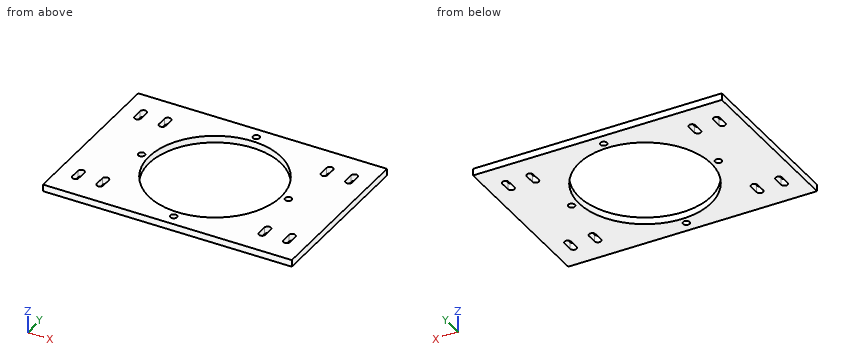
from build123d import *

# Parameters (mm, degrees)
SKETCH1_W                                = 152.4
SKETCH1_H                                = 138.176
SKETCH1_R                                = 53.975
BOSS_EXTRUDE1_DEPTH                      = 5.588
SKETCH5_R                                = 2.665
CUT_EXTRUDE4_DEPTH                       = 450.319819698
CUT_EXTRUDE5_DEPTH                       = 104.008822379
MIRROR1_AT_THE_SECOND_PLANE_COPY_1_DEPTH = 104.008822379
SKETCH7_W                                = 5.588
SKETCH7_H                                = 138.176
BOSS_EXTRUDE2_DEPTH                      = 25.4
CUT_EXTRUDE6_DEPTH                       = 123.991615519
MIRROR3_COPY_1_DEPTH                     = 123.991615519
SKETCH9_R                                = 2.7
CUT_EXTRUDE7_DEPTH                       = 483.750396617


with BuildPart() as part:
    # Sketch1 → Boss-Extrude1 (new body)
    with BuildSketch(Plane.XY):
        Rectangle(SKETCH1_W, SKETCH1_H)
        Circle(SKETCH1_R, mode=Mode.SUBTRACT)
    extrude(amount=BOSS_EXTRUDE1_DEPTH)

    # Sketch5 → Cut-Extrude4 (cut, through all)
    with BuildSketch(Plane(origin=(-338.200209725, -104.490630048, 5.588), x_dir=(0.9999190535665993, -0.012723455288419956, 0), z_dir=(0, 0, 1))):
        with Locations(Location((403.626134832, 63.40628164, 0), (0, 0, 0.729019959))):
            Circle(SKETCH5_R)
    extrude(amount=-CUT_EXTRUDE4_DEPTH, mode=Mode.SUBTRACT)

    # Sketch6 → Cut-Extrude5 (cut, through all)
    with BuildSketch(Plane(origin=(0, 0, 0), x_dir=(-1, 0, 0), z_dir=(0, 0, -1))):
        with BuildLine():
            Line((-68.865, -49.163584611), (-68.865, -41.163584611))
            ThreePointArc((-68.865, -41.163584611), (-66.2, -38.498584611), (-63.535, -41.163584611))
            Line((-63.535, -41.163584611), (-63.535, -49.163584611))
            ThreePointArc((-63.535, -49.163584611), (-66.2, -51.828584611), (-68.865, -49.163584611))
        make_face()
    cut_extrude5 = extrude(amount=-CUT_EXTRUDE5_DEPTH, mode=Mode.SUBTRACT)

    # Mirror1: Cut-Extrude5 across plane
    add(cut_extrude5.mirror(Plane(origin=(0, 0, 0), x_dir=(0, 0, 1), z_dir=(1, 0, 0))), mode=Mode.SUBTRACT)

    # Mirror1 at the second plane: Cut-Extrude5 across plane
    add(cut_extrude5.mirror(Plane.ZX), mode=Mode.SUBTRACT)

    # Mirror1 at the second plane copy 1 sketc → Mirror1 at the second plane copy 1 (cut, through all)
    with BuildSketch(Plane(origin=(0, 0, 0), x_dir=(1, 0, 0), z_dir=(0, 0, -1))):
        with BuildLine():
            Line((-68.865, -49.163584611), (-68.865, -41.163584611))
            ThreePointArc((-68.865, -41.163584611), (-66.2, -38.498584611), (-63.535, -41.163584611))
            Line((-63.535, -41.163584611), (-63.535, -49.163584611))
            ThreePointArc((-63.535, -49.163584611), (-66.2, -51.828584611), (-68.865, -49.163584611))
        make_face()
    extrude(amount=-MIRROR1_AT_THE_SECOND_PLANE_COPY_1_DEPTH, mode=Mode.SUBTRACT)

    # Sketch7 → Boss-Extrude2 (add)
    with BuildSketch(Plane(origin=(76.2, 0, 0), x_dir=(0, 0, -1), z_dir=(1, 0, 0))):
        with Locations((-2.794, 0)):
            Rectangle(SKETCH7_W, SKETCH7_H)
    boss_extrude2 = extrude(amount=BOSS_EXTRUDE2_DEPTH)

    # Sketch8 → Cut-Extrude6 (cut, through all)
    with BuildSketch(Plane(origin=(0, 0, 0), x_dir=(-1, 0, 0), z_dir=(0, 0, -1))):
        with BuildLine():
            Line((-63.535, 49.163584611), (-63.535, 41.163584611))
            ThreePointArc((-63.535, 41.163584611), (-66.2, 38.498584611), (-68.865, 41.163584611))
            Line((-68.865, 41.163584611), (-68.865, 49.163584611))
            ThreePointArc((-68.865, 49.163584611), (-66.2, 51.828584611), (-63.535, 49.163584611))
        make_face()
        with BuildLine():
            Line((-83.535, 41.163584611), (-83.535, 49.163584611))
            ThreePointArc((-83.535, 49.163584611), (-86.2, 51.828584611), (-88.865, 49.163584611))
            Line((-88.865, 49.163584611), (-88.865, 41.163584611))
            ThreePointArc((-88.865, 41.163584611), (-86.2, 38.498584611), (-83.535, 41.163584611))
        make_face()
    cut_extrude6 = extrude(amount=-CUT_EXTRUDE6_DEPTH, mode=Mode.SUBTRACT)

    # Mirror2: Cut-Extrude6 across plane
    add(cut_extrude6.mirror(Plane.ZX), mode=Mode.SUBTRACT)

    # Mirror3: Boss-Extrude2, Cut-Extrude6 across plane
    add(boss_extrude2.mirror(Plane(origin=(0, 0, 0), x_dir=(0, 0, 1), z_dir=(1, 0, 0))))
    add(cut_extrude6.mirror(Plane(origin=(0, 0, 0), x_dir=(0, 0, 1), z_dir=(1, 0, 0))), mode=Mode.SUBTRACT)

    # Mirror3 copy 1 sketch → Mirror3 copy 1 (cut, through all)
    with BuildSketch(Plane(origin=(0, 0, 0), x_dir=(1, 0, 0), z_dir=(0, 0, -1))):
        with BuildLine():
            Line((-63.535, 49.163584611), (-63.535, 41.163584611))
            ThreePointArc((-63.535, 41.163584611), (-66.2, 38.498584611), (-68.865, 41.163584611))
            Line((-68.865, 41.163584611), (-68.865, 49.163584611))
            ThreePointArc((-68.865, 49.163584611), (-66.2, 51.828584611), (-63.535, 49.163584611))
        make_face()
        with BuildLine():
            Line((-83.535, 41.163584611), (-83.535, 49.163584611))
            ThreePointArc((-83.535, 49.163584611), (-86.2, 51.828584611), (-88.865, 49.163584611))
            Line((-88.865, 49.163584611), (-88.865, 41.163584611))
            ThreePointArc((-88.865, 41.163584611), (-86.2, 38.498584611), (-83.535, 41.163584611))
        make_face()
    extrude(amount=-MIRROR3_COPY_1_DEPTH, mode=Mode.SUBTRACT)

    # Sketch9 → Cut-Extrude7 (cut, through all)
    with BuildSketch(Plane(origin=(-338.200209725, -129.890630048, 0), x_dir=(-0.9999190535665993, 0.012723455288419956, 0), z_dir=(0, 0, -1))):
        with Locations(Location((-276.525032787, 133.419783795, 0), (0, 0, 359.270980041))):
            Circle(SKETCH9_R)
        with Locations(Location((-337.283583318, 74.188047898, 0), (0, 0, 359.270980041))):
            Circle(SKETCH9_R)
        with Locations(Location((-396.515319215, 134.946598429, 0), (0, 0, 359.270980041))):
            Circle(SKETCH9_R)
        with Locations(Location((-335.756768683, 194.178334326, 0), (0, 0, 359.270980041))):
            Circle(SKETCH9_R)
    extrude(amount=-CUT_EXTRUDE7_DEPTH, mode=Mode.SUBTRACT)


solid = part.part
Verification items for the finished model (mm, model axes). Coordinates: 2 decimals unless noted, no trailing zeros. Loops run counter-clockwise (first coordinate to the right, second up) from the corner with the lowest first, then second, coordinate; pieces in that order, holes last. Notation, with made-up numbers: (5, 80) -> (34, 80) arc R24 ccw to (34, 95) -> close; hole circle Ø6 at (70.25, 6). An arc over 180 degrees is marked (long way). Answer as CSV lines item,"result".
1) Cross-section at B-B, the plane y = -60. Record the cut outline in (x, z), then the cut area to 3 significant figures.
Found:
outline,"(-101.6, 0) -> (-2.7, 0) -> (-2.7, 5.59) -> (-101.6, 5.59) -> close; (2.7, 0) -> (101.6, 0) -> (101.6, 5.59) -> (2.7, 5.59) -> close"
area,"1,110 mm2"
2) Cross-section at D-D, the plane y = 0. Record the cut outline in (x, z) (3 decimals).
Found:
outline,"(-101.6, 0) -> (-62.7, 0) -> (-62.7, 5.588) -> (-101.6, 5.588) -> close; (-57.3, 0) -> (-53.975, 0) -> (-53.975, 5.588) -> (-57.3, 5.588) -> close; (53.975, 0) -> (57.3, 0) -> (57.3, 5.588) -> (53.975, 5.588) -> close; (62.7, 0) -> (101.6, 0) -> (101.6, 5.588) -> (62.7, 5.588) -> close"
3) Cross-section at A-A, the plane x = 0. Record the cut outline in (y, z) (3 decimals), then the cut area to 3 significant figures.
Found:
outline,"(-69.088, 0) -> (-62.7, 0) -> (-62.7, 5.588) -> (-69.088, 5.588) -> close; (-57.3, 0) -> (-53.975, 0) -> (-53.975, 5.588) -> (-57.3, 5.588) -> close; (53.975, 0) -> (57.3, 0) -> (57.3, 5.588) -> (53.975, 5.588) -> close; (62.7, 0) -> (69.088, 0) -> (69.088, 5.588) -> (62.7, 5.588) -> close"
area,"109 mm2"
4) Cross-section at C-C, the plane x = -66.2. Record the cut outline in (y, z), then the cut area to 3 significant figures.
Found:
outline,"(-69.09, 0) -> (-51.83, 0) -> (-51.83, 5.59) -> (-69.09, 5.59) -> close; (-38.5, 0) -> (38.5, 0) -> (38.5, 5.59) -> (-38.5, 5.59) -> close; (51.83, 0) -> (69.09, 0) -> (69.09, 5.59) -> (51.83, 5.59) -> close"
area,"623 mm2"
5) Thickness scan on L1, parallel to Y at x = 0, z = 4.4 (3 decimals); L2, parallel to Y at x = 65, z = 2.75; L3, parallel to Y at x = -85.5, z = 2.3 (3 decimals). Record the ranges inside material, lowest first. Write a range as from..to.
Found:
L1,"y = -69.088..-62.7, -57.3..-53.975, 53.975..57.3, 62.7..69.088"
L2,"y = -69.09..-51.54, -38.78..38.78, 51.54..69.09"
L3,"y = -69.088..-51.735, -38.592..38.592, 51.735..69.088"
